from build123d import *

# Parameters (mm, degrees)
SKETCH_1_R      = 11
SKETCH_1_R_2    = 2.2
EXTRUDE_1_DEPTH = 2


with BuildPart() as part:
    # 草图1 → 凸台-拉伸1 (new body)
    with BuildSketch(Plane(origin=(0, 0, 0), x_dir=(1, 0, 0), z_dir=(0, 1, 0))):
        Polygon((159.754738648, 48.995603023), (150.004738648, 48.995603023), (150.004738648, 46.495603023), (151.504738648, 46.495603023), (151.504738648, 43.895603023), (150.004738648, 43.895603023), (150.004738648, 40.895603023), (147.004738648, 40.895603023), (147.004738648, 43.895603023), (145.504738648, 43.895603023), (145.504738648, 46.495603023), (147.004738648, 46.495603023), (147.004738648, 48.995603023), (138.604738648, 48.995603023), (133.504738648, 48.995603023), (118.504738648, 48.995603023), (118.504738648, 33.995603023), (118.504738648, 21.495603023), (118.504738648, 20.495603023), (121.004738648, 20.495603023), (121.004738648, 21.995603023), (123.604738648, 21.995603023), (123.604738648, 20.495603023), (126.604738648, 20.495603023), (126.604738648, 17.495603023), (123.604738648, 17.495603023), (123.604738648, 15.995603023), (121.004738648, 15.995603023), (121.004738648, 17.495603023), (118.504738648, 17.495603023), (118.504738648, 7.745603023), (116.504738648, 7.745603023), (116.504738648, -0.254396977), (118.504738648, -0.254396977), (118.504738648, -27.754396977), (116.504738648, -27.754396977), (116.504738648, -35.754396977), (118.504738648, -35.754396977), (118.504738648, -45.504396977), (121.004738648, -45.504396977), (121.004738648, -44.004396977), (123.604738648, -44.004396977), (123.604738648, -45.504396977), (126.604738648, -45.504396977), (126.604738648, -48.504396977), (123.604738648, -48.504396977), (123.604738648, -50.004396977), (121.004738648, -50.004396977), (121.004738648, -48.504396977), (118.504738648, -48.504396977), (118.504738648, -56.904396977), (118.504738648, -62.004396977), (118.504738648, -77.004396977), (133.504738648, -77.004396977), (146.004738648, -77.004396977), (147.004738648, -77.004396977), (147.004738648, -74.504396977), (145.504738648, -74.504396977), (145.504738648, -71.904396977), (147.004738648, -71.904396977), (147.004738648, -68.904396977), (150.004738648, -68.904396977), (150.004738648, -71.904396977), (151.504738648, -71.904396977), (151.504738648, -74.504396977), (150.004738648, -74.504396977), (150.004738648, -77.004396977), (159.754738648, -77.004396977), (159.754738648, -79.004396977), (167.754738648, -79.004396977), (167.754738648, -77.004396977), (195.254738648, -77.004396977), (195.254738648, -79.004396977), (203.254738648, -79.004396977), (203.254738648, -77.004396977), (213.004738648, -77.004396977), (213.004738648, -74.504396977), (211.504738648, -74.504396977), (211.504738648, -71.904396977), (213.004738648, -71.904396977), (213.004738648, -68.904396977), (216.004738648, -68.904396977), (216.004738648, -71.904396977), (217.504738648, -71.904396977), (217.504738648, -74.504396977), (216.004738648, -74.504396977), (216.004738648, -77.004396977), (224.404738648, -77.004396977), (229.504738648, -77.004396977), (244.504738648, -77.004396977), (244.504738648, -62.004396977), (244.504738648, -49.504396977), (244.504738648, -48.504396977), (242.004738648, -48.504396977), (242.004738648, -50.004396977), (239.404738648, -50.004396977), (239.404738648, -48.504396977), (236.404738648, -48.504396977), (236.404738648, -45.504396977), (239.404738648, -45.504396977), (239.404738648, -44.004396977), (242.004738648, -44.004396977), (242.004738648, -45.504396977), (244.504738648, -45.504396977), (244.504738648, -35.754396977), (246.504738648, -35.754396977), (246.504738648, -27.754396977), (244.504738648, -27.754396977), (244.504738648, -0.254396977), (246.504738648, -0.254396977), (246.504738648, 7.745603023), (244.504738648, 7.745603023), (244.504738648, 17.495603023), (242.004738648, 17.495603023), (242.004738648, 15.995603023), (239.404738648, 15.995603023), (239.404738648, 17.495603023), (236.404738648, 17.495603023), (236.404738648, 20.495603023), (239.404738648, 20.495603023), (239.404738648, 21.995603023), (242.004738648, 21.995603023), (242.004738648, 20.495603023), (244.504738648, 20.495603023), (244.504738648, 28.895603023), (244.504738648, 33.995603023), (244.504738648, 48.995603023), (229.504738648, 48.995603023), (217.004738648, 48.995603023), (216.004738648, 48.995603023), (216.004738648, 46.495603023), (217.504738648, 46.495603023), (217.504738648, 43.895603023), (216.004738648, 43.895603023), (216.004738648, 40.895603023), (213.004738648, 40.895603023), (213.004738648, 43.895603023), (211.504738648, 43.895603023), (211.504738648, 46.495603023), (213.004738648, 46.495603023), (213.004738648, 48.995603023), (203.254738648, 48.995603023), (203.254738648, 50.995603023), (195.254738648, 50.995603023), (195.254738648, 48.995603023), (167.754738648, 48.995603023), (167.754738648, 50.995603023), (159.754738648, 50.995603023), align=None)
        with Locations(Location((181.504738648, -14.004396977, 0), (0, 0, 270))):
            Circle(SKETCH_1_R, mode=Mode.SUBTRACT)
        with Locations(Location((181.504738648, -36.004396977, 0), (0, 0, 270))):
            Circle(SKETCH_1_R_2, mode=Mode.SUBTRACT)
        with Locations(Location((159.504738648, -14.004396977, 0), (0, 0, 270))):
            Circle(SKETCH_1_R_2, mode=Mode.SUBTRACT)
        with Locations(Location((181.504738648, 7.995603023, 0), (0, 0, 270))):
            Circle(SKETCH_1_R_2, mode=Mode.SUBTRACT)
        with Locations(Location((203.504738648, -14.004396977, 0), (0, 0, 270))):
            Circle(SKETCH_1_R_2, mode=Mode.SUBTRACT)
    extrude(amount=EXTRUDE_1_DEPTH)


solid = part.part
Input: part model. Units: mm. Frame: model coordinates. Coordinates: 2 decimals unless noted, no trailing zeros. Loops run counter-clockwise (first coordinate to the right, second up) from the corner with the lowest first, then second, coordinate; pieces in that order, holes last.
(1) Pull-direction query (X, two-part tool) for faces 1 (the face through (201.553, 0.986, 15.02)), 2 (the face through (195, 2, 13)); classes: released by +X, released by -X, zero draft, split by the parting line, or undercut.
(2) Material intervals for probe 1 along Z at (x, y) = (237, 0.4); probe 2 along X at (y, z) = (0.2, 13.5); probe 3 along X at (y, z) = (1.7, 26.5), sorted ascending.
(3) Section D-D on y = 1.5. Count the separate pieces of the cut face and the enclosed holes in it, then the cut area to 3 significant figures.
(4) First-contact query: pin 1 Ø1 at (y, z) = (1.5, 78) entering from -X; pin 2 Ø10 at (x, z) = (190.5, 37) entering from -Y; pin 3 Ø0.6 at (x, y) = (245.5, 1) entering from +Z; pin 4 Ø0.6 at (x, y) = (179, 1) entering from +Z. Flat tips, straight axial feed; report the tip coordinate or a pass-through.
(5) Section A-A on x = 173. Return the cut outline in (y, z).
(6) Section B-B on z = 13.5. Return the cut outline in (x, y).
(7) Section C-C on z = -28.5. Return the cut outline in (x, y).
Data:
1. face 1: undercut
1. face 2: zero draft
2. probe 1: z = -49 to -20.5, -17.5 to 45.5, 48.5 to 77
2. probe 2: x = 118.5 to 157.36, 161.65 to 170.52, 192.49 to 201.36, 205.65 to 244.5
2. probe 3: x = 118.5 to 244.5
3. separate pieces: 1
3. enclosed holes: 5
3. area: 15,300 mm2
4. pin 1: stops at x = 159.75
4. pin 2: stops at y = 0
4. pin 3: stops at z = 35.75
4. pin 4: stops at z = 77
5. outline: (0, -49) - (2, -49) - (2, 7.03) - (0, 7.03) - close; (0, 20.98) - (2, 20.98) - (2, 77) - (0, 77) - close
6. outline: (118.5, 0) - (157.36, 0) - (157.36, 2) - (118.5, 2) - close; (161.65, 0) - (170.52, 0) - (170.52, 2) - (161.65, 2) - close; (192.49, 0) - (201.36, 0) - (201.36, 2) - (192.49, 2) - close; (205.65, 0) - (244.5, 0) - (244.5, 2) - (205.65, 2) - close
7. outline: (118.5, 0) - (244.5, 0) - (244.5, 2) - (118.5, 2) - close
